Could you check a few things on this model? Use its own coordinates, in mm. Face numbers are marked on the shaded views. A direction names the side the tool comes from. Give positions to 0.01 mm unless a question says otherwise; leave off trailing zeros. Loops run counter-clockwise (first coordinate to the right, second up) from the corner with the lowest first, then second, coordinate; pieces in that order, holes last. Notation, with made-up numbers: (48.5, -24.5) - (61.5, -24.5) arc R36 cw to (61.5, 11.5) - close; hole circle Ø10 at (34, 43). An arc over 180 degrees is marked (long way). Use CSV: the item, a comma, the result in double quotes.
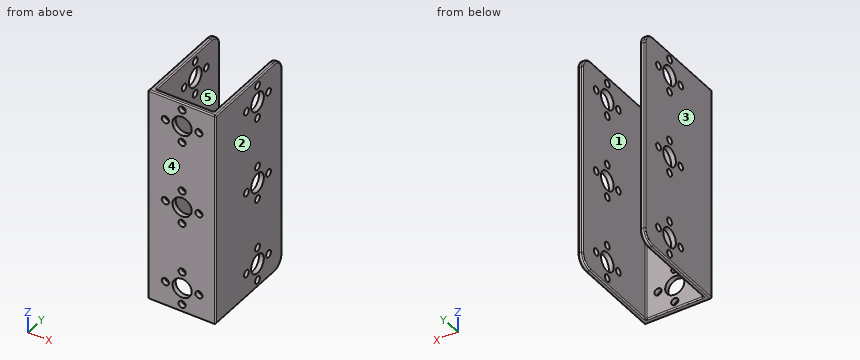
from build123d import *

# Parameters (mm, degrees)
SKETCH1_W                 = 28
SKETCH1_H                 = 90
BOSS_EXTRUDE1_DEPTH       = 2
SKETCH2_W                 = 2
SKETCH2_H                 = 90
BOSS_EXTRUDE2_DEPTH       = 40
FILLET2_R                 = 5
FILLET3_R                 = 0.5
F_8_0MM_DOWEL_HOLE1_D     = 8
F_3_0MM_DOWEL_HOLE2_D     = 3
F_8_0MM_DOWEL_HOLE2_D     = 8
F_8_0MM_DOWEL_HOLE2_DEPTH = 3
F_8_0MM_DOWEL_HOLE2_TIP   = 2.403442476
F_3_0MM_DOWEL_HOLE3_D     = 3


with BuildPart() as part:
    # Sketch1 → Boss-Extrude1 (new body)
    with BuildSketch(Plane(origin=(0, 0, 0), x_dir=(1, 0, 0), z_dir=(0, 1, 0))):
        Rectangle(SKETCH1_W, SKETCH1_H)
    extrude(amount=BOSS_EXTRUDE1_DEPTH)

    # Sketch2 → Boss-Extrude2 (add)
    with BuildSketch(Plane(origin=(0, 2, 0), x_dir=(1, 0, 0), z_dir=(0, 1, 0))):
        with Locations((13, 0)):
            Rectangle(SKETCH2_W, SKETCH2_H)
        with Locations((-13, 0)):
            Rectangle(SKETCH2_W, SKETCH2_H)
    extrude(amount=BOSS_EXTRUDE2_DEPTH)

    # Fillet2
    fillet2_edges = [part.edges().sort_by_distance(p)[0] for p in [
        (13, 42, -45),
        (13, 42, 45),
        (-13, 42, 45),
        (-13, 42, -45),
    ]]
    fillet(fillet2_edges, radius=FILLET2_R)

    # Fillet3
    fillet3_edges = [part.edges().sort_by_distance(p)[0] for p in [
        (0, 2, -45),
        (12, 2, 0),
        (0, 2, 45),
        (-12, 2, 0),
        (14, 42, 0),
        (12, 42, 0),
        (12, 19.5, 45),
        (12, 19.5, -45),
        (12, 40.535533906, 43.535533906),
        (12, 40.535533906, -43.535533906),
        (-14, 18.5, -45),
        (-12, 19.5, -45),
        (14, 18.5, -45),
        (14, 18.5, 45),
        (14, 40.535533906, 43.535533906),
        (14, 40.535533906, -43.535533906),
        (-14, 42, 0),
        (0, 0, 45),
        (-12, 42, 0),
        (-14, 18.5, 45),
        (-14, 40.535533906, 43.535533906),
        (-14, 40.535533906, -43.535533906),
        (-12, 19.5, 45),
        (-12, 40.535533906, 43.535533906),
        (-12, 40.535533906, -43.535533906),
        (14, 0, 0),
    ]]
    fillet(fillet3_edges, radius=FILLET3_R)

    # Ø8.0mm Dowel Hole1 (through all)
    with Locations(Plane(origin=(14, 0, 0), x_dir=(0, 0, -1), z_dir=(1, 0, 0))):
        with Locations((0, 26.5), (-35, 26.5), (35, 26.5)):
            Hole(F_8_0MM_DOWEL_HOLE1_D / 2)

    # Ø3.0mm Dowel Hole2 (through all)
    with Locations(Plane(origin=(14, 0, 0), x_dir=(0, 0, -1), z_dir=(1, 0, 0))):
        with Locations((-35, 33.5), (-28, 26.5), (-35, 19.5), (-42, 26.5), (-35, 26.5), (0, 33.5), (7, 26.5), (0, 19.5), (-7, 26.5), (35, 33.5), (42, 26.5), (35, 19.5), (28, 26.5), (0, 26.5), (35, 26.5)):
            Hole(F_3_0MM_DOWEL_HOLE2_D / 2)

    # Ø8.0mm Dowel Hole2
    with Locations(Plane(origin=(0, 0, 0), x_dir=(-1, 0, 0), z_dir=(0, -1, 0))):
        with Locations((0, 0), (0, 35), (0, -35)):
            Hole(F_8_0MM_DOWEL_HOLE2_D / 2, depth=F_8_0MM_DOWEL_HOLE2_DEPTH)
            with Locations((0, 0, -(F_8_0MM_DOWEL_HOLE2_DEPTH + F_8_0MM_DOWEL_HOLE2_TIP / 2))):  # 118° drill point
                Cone(0, F_8_0MM_DOWEL_HOLE2_D / 2, F_8_0MM_DOWEL_HOLE2_TIP, mode=Mode.SUBTRACT)

    # Ø3.0mm Dowel Hole3 (through all)
    with Locations(Plane(origin=(0, 0, 0), x_dir=(-1, 0, 0), z_dir=(0, -1, 0))):
        with Locations((0, -7), (0, -35), (0, -28), (0, 35), (0, 28), (7, 0), (0, 7), (-7, 0), (0, 0), (7, -35), (0, -42), (-7, -35), (-7, 35), (0, 42), (7, 35)):
            Hole(F_3_0MM_DOWEL_HOLE3_D / 2)


solid = part.part
1) Suppose I cut it at D-D (x = 0). State how many separate pieces and enclosed holes the cut face has, plus the area to 3 significant figures.
Answer below:
separate pieces,"10"
enclosed holes,"0"
area,"95.8 mm2"
2) I need wall thicknesses on line 1 along Z through (x, y) = (-7, 0.95); line 2 along X through (y, z) = (30, -5.5); line 3 along Y through (x, z) = (-13.45, -28). Which ranges of each line are inside material? Lowest first, please.
Answer below:
line 1,"z = -45 to -36.5, -33.5 to -1.5, 1.5 to 33.5, 36.5 to 45"
line 2,"x = -14 to -12, 12 to 14"
line 3,"y = 0 to 25, 28 to 42"
3) Suppose I cut it at C-C (x = -7). Please give me the cut outline in (y, z).
Answer below:
outline,"(0, -45) - (1.5, -45) arc R0.5 ccw to (2, -44.5) - (2, -36.5) - (0, -36.5) - close; (0, -33.5) - (2, -33.5) - (2, -1.5) - (0, -1.5) - close; (0, 1.5) - (2, 1.5) - (2, 33.5) - (0, 33.5) - close; (0, 36.5) - (2, 36.5) - (2, 44.5) arc R0.5 ccw to (1.5, 45) - (0.5, 45) arc R0.5 ccw to (0, 44.5) - close"
4) I'm going to push a flat-ended pin straight in: P1, Ø4, axis at x = 7, z = -35, coming from the +Y side. Where does the tip first touch, or does it pass through?
Answer below:
P1,"stops at y = 2"
5) We'd pull the mould along X, two halves only. Please class the marked faces 3, 4 and 5: +X half, -X half, draft (parallel to the pull), parting line (faces both ways), or undercut.
Answer below:
face 3,"-X half"
face 4,"draft"
face 5,"undercut"
6) Which directions (+Z, -Z, +X, -X, +Y, -Y) give clear straight access to the entire face, cutting with the end or side of a thin tool? Please do the marked faces 1 and 2.
Answer below:
face 1,"+Z, -Z, +Y"
face 2,"+Z, -Z, +X, +Y, -Y"
7) Suppose I cut it at B-B (z = -28). Please give me the cut outline in (x, y), plus the area to 3 significant figures.
Answer below:
outline,"(-14, 0) - (-1.5, 0) - (-1.5, 2) - (-11.5, 2) arc R0.5 cw to (-12, 2.5) - (-12, 25) - (-14, 25) - close; (-14, 28) - (-12, 28) - (-12, 41.5) arc R0.5 ccw to (-12.5, 42) - (-13.5, 42) arc R0.5 ccw to (-14, 41.5) - close; (1.5, 0) - (13.5, 0) arc R0.5 ccw to (14, 0.5) - (14, 25) - (12, 25) - (12, 2.5) arc R0.5 cw to (11.5, 2) - (1.5, 2) - close; (12, 28) - (14, 28) - (14, 41.5) arc R0.5 ccw to (13.5, 42) - (12.5, 42) arc R0.5 ccw to (12, 41.5) - close"
area,"198 mm2"
8) Suppose I cut it at A-A (y = 9.5). Please give me the cut outline in (x, z), plus the area to 3 significant figures.
Answer below:
outline,"(-14, -44.5) arc R0.5 ccw to (-13.5, -45) - (-12.5, -45) arc R0.5 ccw to (-12, -44.5) - (-12, 44.5) arc R0.5 ccw to (-12.5, 45) - (-13.5, 45) arc R0.5 ccw to (-14, 44.5) - close; (12, -44.5) arc R0.5 ccw to (12.5, -45) - (13.5, -45) arc R0.5 ccw to (14, -44.5) - (14, 44.5) arc R0.5 ccw to (13.5, 45) - (12.5, 45) arc R0.5 ccw to (12, 44.5) - close"
area,"360 mm2"
